Geometry: final body of the model. Coordinates: model frame, mm. A direction names the side the tool comes from. Coordinates: 2 decimals unless noted, no trailing zeros. Order: outer loops, then holes, each group sorted by start corner. A loop starts at its lowest first (then second) coordinate and runs counter-clockwise, first axis right, second up. Notation, with made-up numbers: (26, 80) -> (68, 80) arc R7 ccw to (68, 92) -> close; hole circle Ø10 at (83.5, 25.5). An arc over 180 degrees is marked (long way). Use one line per item in the form item = value.
```python
from build123d import *

# Parameters (mm, degrees)
SKETCH1_W           = 20
SKETCH1_H           = 10.2
SKETCH1_R           = 1.2
BOSS_EXTRUDE1_DEPTH = 6.4
BOSS_EXTRUDE2_DEPTH = 2.5
FILLET1_R           = 0.5


with BuildPart() as part:
    # Sketch1 → Boss-Extrude1 (new body)
    with BuildSketch(Plane(origin=(0, 0, 0), x_dir=(1, 0, 0), z_dir=(0, 1, 0))):
        Rectangle(SKETCH1_W, SKETCH1_H)
        with Locations(Location((-4.75, -2.2, 0), (0, 0, 270))):
            Circle(SKETCH1_R, mode=Mode.SUBTRACT)
        with Locations(Location((4.75, -2.2, 0), (0, 0, 270))):
            Circle(SKETCH1_R, mode=Mode.SUBTRACT)
    extrude(amount=BOSS_EXTRUDE1_DEPTH)

    # Sketch4 → Boss-Extrude2 (add, symmetric)
    with BuildSketch(Plane(origin=(0, 3.2, 0), x_dir=(1, 0, 0), z_dir=(0, 1, 0))):
        with BuildLine():
            Line((-6.75, 5.1), (-6.75, 5.5))
            Line((-6.75, 5.5), (9.55, 5.5))
            ThreePointArc((9.55, 5.5), (10.645445115, 10.03541565), (7.600641131, 6.5))
            Line((7.600641131, 6.5), (-7.75, 6.5))
            Line((-7.75, 6.5), (-7.75, 5.1))
            Line((-7.75, 5.1), (-6.75, 5.1))
        make_face()
    extrude(amount=BOSS_EXTRUDE2_DEPTH, both=True)

    # Fillet1
    # the kernel refuses this fillet: 0.5 mm, written as the material it adds along each edge
    with BuildSketch(Plane(origin=(-6.75, 0.7, -5.5), x_dir=(1.5765166949672097e-12, 0, 1.0), z_dir=(0, 1, 0))) as fillet1_piece_1:
        with BuildLine():
            CenterArc((0.5, 0.489897949), FILLET1_R, 180, 78.463040967)
            Line((0, 0.489897949), (0, 0))
            Line((0, 0), (0.4, 0))
        make_face()
    extrude(amount=5)
    # the kernel refuses this fillet: 0.5 mm, written as the material it takes off along each edge
    with BuildSketch(Plane(origin=(-7.75, 6.95, -6.5), x_dir=(0, 0, 1), z_dir=(0, -1, 0))) as fillet1_2_piece_1:
        with BuildLine():
            CenterArc((FILLET1_R, -FILLET1_R), FILLET1_R, 90, 90)
            Line((0, -FILLET1_R), (0, 0))
            Line((0, 0), (FILLET1_R, 0))
        make_face()
    extrude(amount=7.5, mode=Mode.SUBTRACT)


solid = part.part
```
1) Material intervals for probe 1 along X at (y, z) = (1.5, 2.2); probe 2 along Z at (x, y) = (0.25, 4.5); probe 3 along X at (y, z) = (2, -4.25), sorted ascending. Write a range as from..to.
Results found:
probe_1 = -10..-5.95, -3.55..3.55, 5.95..10
probe_2 = -6.5..-5.5, -5.1..5.1
probe_3 = -10..10
2) Section C-C, the plane y = 4.5. Output: boundary loops of the cut face in (x, z), and give its area (3 significant figures).
Results found:
outline = (-10, -5.1) -> (-7.75, -5.1) -> (-7.75, -6) arc R0.5 ccw to (-7.25, -6.5) -> (7.6, -6.5) arc R2.4 ccw (long way) to (9.55, -5.5) -> (-6.26, -5.5) arc R0.5 cw to (-6.75, -5.1) -> (10, -5.1) -> (10, 5.1) -> (-10, 5.1) -> close; hole circle Ø2.4 at (-4.75, 2.2); hole circle Ø2.4 at (4.75, 2.2)
area = 229 mm2
3) Section A-A, the plane x = -4.75. Output: boundary loops of the cut face in (y, z).
Results found:
outline = (0, -5.1) -> (6.4, -5.1) -> (6.4, 1) -> (0, 1) -> close; (0, 3.4) -> (6.4, 3.4) -> (6.4, 5.1) -> (0, 5.1) -> close; (0.7, -6.5) -> (5.7, -6.5) -> (5.7, -5.5) -> (0.7, -5.5) -> close
4) Contact query for flat-ended pins moving along their axis: P1, Ø3, axis at x = -4.75, z = 2.2, coming from the -Y side; P2, Ø3, axis at y = 4, z = 0, coming from the +X side; P3, Ø1, axis at x = 8.5, z = -8.5, coming from the +Y side; P4, Ø3, axis at x = -2.5, y = 4, coming from the -Z side. Output: stop coordinate, or through.
Results found:
P1 = 0
P2 = 10
P3 = 5.7
P4 = -6.5
5) Pull-direction query (Z, two-part tool) for faces 4 (the flat face through (0, 3, 5.1)), 5 (the cylindrical face through (-4.39, 3.155, 3.345)), 6 (the flat face through (-10, 3, 0)); classes: released by +Z, released by -Z, zero draft, split by the parting line, or undercut.
Results found:
face_4 = released by +Z
face_5 = undercut
face_6 = zero draft
6) Section B-B, the plane z = 2.2. Output: boundary loops of the cut face in (x, y), and give its area (3 significant figures).
Results found:
outline = (-10, 0) -> (-5.95, 0) -> (-5.95, 6.4) -> (-10, 6.4) -> close; (-3.55, 0) -> (3.55, 0) -> (3.55, 6.4) -> (-3.55, 6.4) -> close; (5.95, 0) -> (10, 0) -> (10, 6.4) -> (5.95, 6.4) -> close
area = 97.3 mm2
7) Section D-D, the plane x = 6.25. Output: boundary loops of the cut face in (y, z).
Results found:
outline = (0, -5.1) -> (6.4, -5.1) -> (6.4, 5.1) -> (0, 5.1) -> close; (0.7, -6.5) -> (5.7, -6.5) -> (5.7, -5.5) -> (0.7, -5.5) -> close
8) Access query for faces 1 (the flat face through (6, 0.7, -6)), 2 (the flat face through (6, 5.7, -6)), 3 (the flat face through (10, 3, 0)). Directions: +Z, -Z, +X, -X, +Y, -Y. A direction counts if a zero-diameter tool reaches every point of the face in a straight line with its end or side. Return the directions, or none.
Results found:
face_1 = -Z, +X, -X, -Y
face_2 = -Z, +X, -X, +Y
face_3 = +Z, +X, +Y, -Y
